Could you check a few things on this model? Use its own coordinates, in mm. Coordinates: 2 decimals unless noted, no trailing zeros. Loops run counter-clockwise (first coordinate to the right, second up) from the corner with the lowest first, then second, coordinate; pieces in that order, holes last. Notation, with made-up numbers: M 53,35 L 95,35 A25 ccw 95,68 Z; hole C 48,43 d5. An arc over 180 degrees is marked long. Write each question's results on one line, items separated by ' | '.
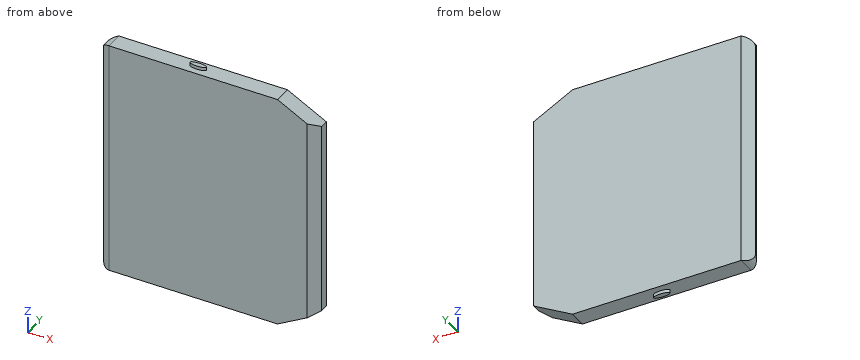
Autodesk Inventor part; units mm, degrees
ref_plane "YZ Plane" through (0, 0, 0) normal (1, 0, 0) x (0, 1, 0)
ref_plane "XZ Plane" through (0, 0, 0) normal (0, 1, 0) x (-1, 0, 0)
ref_plane "XY Plane" through (0, 0, 0) normal (0, 0, 1) x (1, 0, 0)
sketch "Sketch1" plane through (0, 0, 0) normal (0, 1, 0) x (-1, 0, 0)
  line L0 (67.8505, 69.4133) -> (67.8505, -11.5697)
  line L1 (67.8505, -11.5697) -> (6.8505, -11.5697)
  line L2 (6.8505, -11.5697) -> (-6.5145, -4.1373)
  line L3 (-6.5145, -4.1373) -> (-6.5145, 62.3267)
  line L4 (-6.5145, 62.3267) -> (6.8505, 69.4133)
  line L5 (6.8505, 69.4133) -> (67.8505, 69.4133)
extrude "Extrusion1" add sketch "Sketch1" along normal blind 6
sketch "Sketch2" plane through (-6.8505, 0, -11.5697) normal (0, 0, -1) x (-1, 0, 0)
  line L0 (0, 0) -> (0, 6) construction
  ellipse E0 centre (28.92, 3) end of major axis (31.716, 3) minor radius 0.841
  line L1 (-13.365, 0) -> (-13.365, 6) construction
  point P0 (-6.8505, 0)
  dimension "d9" = 2.796
  dimension "d12" = 0.841
  dimension "d11" = 28.92
extrude "Extrusion2" add sketch "Sketch2" along normal blind 1.125
sketch "Sketch3" plane through (-67.8505, 0, 69.4133) normal (0, 0, 1) x (1, 0, 0)
  ellipse E0 centre (32.08, 3) end of major axis (34.876, 3) minor radius 0.841 construction
  ellipse E1 centre (32.08, 3) end of major axis (29.284, 3) minor radius 0.841
  point P0 (67.8505, 0)
extrude "Extrusion3" add sketch "Sketch3" along normal blind 1.125
chamfer "Chamfer1" distance 3.175 angle 45 1 edges at (-67.8505, 6, 28.9218)
fillet "Fillet1" radius 3.175 3 edges at (-67.8505, 0, 28.9218) (-67.8505, 1.4125, -11.5697) (-67.8505, 1.4125, 69.4133)
chamfer "Chamfer2" distance 3.175 angle 45 1 edges at (6.5145, 0, 29.0947)
properties part number "Moto G3 Phone Case Back"
(1) Will these pins go through, and if not, where does the flat tip stop? P1, Ø2, axis at x = -15.5, y = 2.5, coming from the -Z side; P2, Ø1.8, axis at x = -23.5, y = 3.5, coming from the +Z side; P3, Ø1.5, axis at x = -59.5, z = 25, coming from the -Y side; P4, Ø2, axis at y = 4.5, z = 61, coming from the -X side.
Reported:
P1: stops at z = -11.57 | P2: stops at z = 69.41 | P3: stops at y = 0 | P4: stops at x = -67.18
(2) Imagine slicing it at D-D, the plane x = -2. List the corners of the cut face in (y, z) for me.
Reported:
outline: M 0,-8.87 L 6,-8.87 L 6,66.84 L 0,66.84 Z
(3) Please list where these lines run through material, in increasing order: probe 1 along Z at (x, y) = (-41, 2.75); probe 2 along Y at (x, z) = (3.5, 50.5); probe 3 along X at (y, z) = (5.5, 63). Write a range as from..to.
Reported:
probe 1: z = -11.57..69.41 | probe 2: y = 0.16..6 | probe 3: x = -65.18..5.24
(4) Imagine slicing it at B-B, the plane x = -53.5. List the corners of the cut face in (y, z) for me.
Reported:
outline: M 0,-11.57 L 6,-11.57 L 6,69.41 L 0,69.41 Z
